Could you check a few things on this drawing? It's one solid part, dimensions in mm from its lowest x, y, z. A direction names the side the tool comes from. Coordinates: 2 decimals unless noted, no trailing zeros. Order: outer loops, then holes, each group sorted by start corner. A loop starts at its lowest first (then second) coordinate and runs counter-clockwise, first axis right, second up.
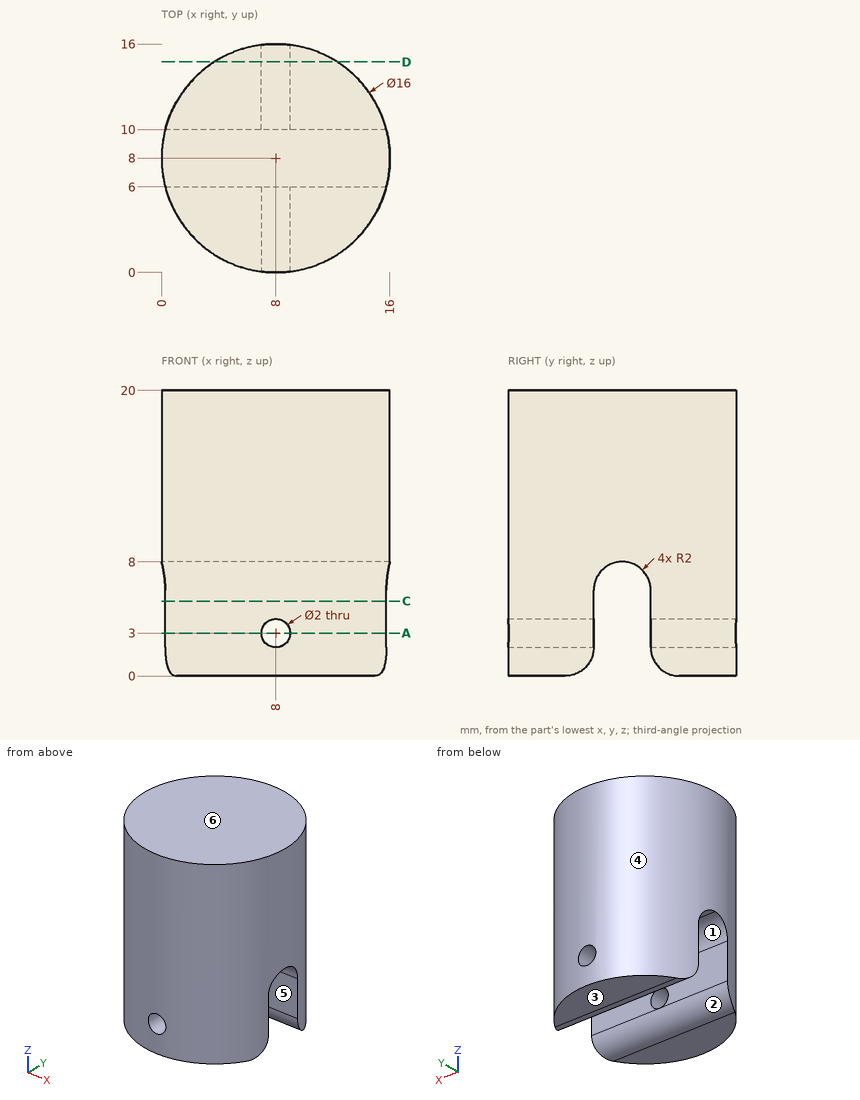
1. Imagine slicing it at D-D on y = 14.75. Please give me the cut outline in (x, z).
Completed:
outline: (3.71, 0) - (12.29, 0) - (12.29, 20) - (3.71, 20) - close; hole circle Ø2 at (8, 3)
2. On a 3-axis mill with a long thin cutter (end or side, diameter ignored), from which of +Z, -Z, +X, -X, +Y, -Y can I reach the whole of each face in a straight line? I mean the marked faces 5 and 6. Say none if no direction works.
Completed:
face 5: -Z, +X, -X
face 6: +Z, +X, -X, +Y, -Y
3. Please list where these lines run through material, in increasing order: probe 1 along Z at (x, y) = (8, 14.75); probe 2 along Y at (x, z) = (8.25, 12.25); probe 3 along Y at (x, z) = (1.75, 4).
Completed:
probe 1: z = 0 to 2, 4 to 20
probe 2: y = 0 to 16
probe 3: y = 3.01 to 6, 10 to 12.99
4. Thinking about a two-plate mould opening in Y: for the marked faces 1, 2, 3 and 4, which applies, pulls with the +Y half, pulls with the -Y half, needs draft (parallel to the pull), parting line crosses it, or undercut?
Completed:
face 1: undercut
face 2: undercut
face 3: needs draft
face 4: parting line crosses it
5. Imagine slicing it at C-C on z = 5.25. Please give me the cut outline in (x, y), then the cut area to 3 significant figures.
Completed:
outline: (0.25, 6) arc R8 ccw to (15.75, 6) - close; (0.25, 10) - (15.75, 10) arc R8 ccw to start
area: 138 mm2
6. I'm going to push flat-ended pins straight in: pin 1 (1 mm diameter, centred on y = 2.5, z = 12, fed in from +X) (3 decimals); pin 2 (6 mm diameter, centred on x = 5.5, y = 7.5, fed in from -Z); pin 3 (6 mm diameter, centred on y = 4, z = 13.5, fed in from -X). Where does each tip first touch, or does it pass through?
Completed:
pin 1: stops at x = 14.245
pin 2: stops at z = 0.06
pin 3: stops at x = 0.06
7. Imagine slicing it at A-A on z = 3. Please give me the cut outline in (x, y).
Completed:
outline: (0.25, 6) arc R8 ccw to (7, 0.06) - (7, 6) - close; (0.25, 10) - (7, 10) - (7, 15.94) arc R8 ccw to start; (9, 0.06) arc R8 ccw to (15.75, 6) - (9, 6) - close; (9, 10) - (15.75, 10) arc R8 ccw to (9, 15.94) - close
